Source: CAD feature listing. Evaluate the final solid. Frame: model axes, mm. Give positions to 0.01 mm unless a question says otherwise; leave off trailing zeros. Loops run counter-clockwise (first coordinate to the right, second up) from the corner with the lowest first, then second, coordinate; pieces in that order, holes last. Notation, with made-up numbers: M -23.5,26 L 11.5,26 A23 cw 11.5,41 Z; hole C -9,60.25 d1. An arc over 180 degrees is marked long. Answer in a Markdown table with one row per item.
```python
from build123d import *

# Parameters (mm, degrees)
F1_DEPTH = 175
F2_R     = 2
F3_DEPTH = 6.001


with BuildPart() as f1:
    # F0 (on Front) → F1 (new body)
    with BuildSketch(Plane.XZ):
        Polygon((4.5, 6), (-4.5, 6), (-4.5, 4.5), (-3.8, 4), (-4.5, 3.5), (-4.5, 0), (4.5, 0), (4.5, 3.5), (3.8, 4), (4.5, 4.5), align=None)
    extrude(amount=F1_DEPTH)

    # F2 (on face) → F3 (cut, through all)
    with BuildSketch(Plane.XY.offset(6)):
        with Locations((0, -7)):
            Circle(F2_R)
        with Locations((0, -27)):
            Circle(F2_R)
        with Locations((0, -47)):
            Circle(F2_R)
        with Locations((0, -67)):
            Circle(F2_R)
        with Locations((0, -87)):
            Circle(F2_R)
        with Locations((0, -107)):
            Circle(F2_R)
        with Locations((0, -127)):
            Circle(F2_R)
        with Locations((0, -147)):
            Circle(F2_R)
        with Locations((0, -167)):
            Circle(F2_R)
    extrude(amount=-F3_DEPTH, mode=Mode.SUBTRACT)


solid = f1.part
```
Q1. Section query A-A (z = 1.8). Give the number of separate pieces and of enclosed holes in the cut face, plus the area to 3 significant figures.
Values follow:
| item | result |
|---|---|
| separate pieces | 1 |
| enclosed holes | 9 |
| area | 1,460 mm^2 |
Q2. Contact query for a flat-ended pin moving along its axis: pin 1 Ø3 at (x, y) = (0, -27) entering from +Z (3 decimals). Output: stop coordinate, or through.
Values follow:
| item | result |
|---|---|
| pin 1 | through |
Q3. Section query B-B (y = -87). Output: boundary loops of the cut face in (x, z), plus the area to 3 significant figures.
Values follow:
| item | result |
|---|---|
| outline | M -4.5,0 L -2,0 L -2,6 L -4.5,6 L -4.5,4.5 L -3.8,4 L -4.5,3.5 Z; M 2,0 L 4.5,0 L 4.5,3.5 L 3.8,4 L 4.5,4.5 L 4.5,6 L 2,6 Z |
| area | 29.3 mm^2 |
Q4. Ray query, probe 1 along X at (y, z) = (-167, 4.75); probe 2 along Z at (x, y) = (-4, -149); probe 3 along X at (y, z) = (-125.5, 2.6). Return the intervals inside material, ascending. Write a range as from..to.
Values follow:
| item | result |
|---|---|
| probe 1 | -4.5..-2, 2..4.5 |
| probe 2 | 0..3.86, 4.14..6 |
| probe 3 | -4.5..-1.32, 1.32..4.5 |
Q5. Mould query, pull axis Y, two halves, no side actions, for faces 1 (the flat face through (-4.5, -86, 2)), 2 (the cylindrical face through (0.923, -168.774, 3.042)), 3 (the flat face through (0, 0, 3)). Classes: +Y half, -Y half, draft (parallel to the pull), parting line (faces both ways), or undercut.
Values follow:
| item | result |
|---|---|
| face 1 | draft |
| face 2 | undercut |
| face 3 | +Y half |
